The listing builds one solid part. Answer for the finished solid, in the listing's coordinates (mm). A direction names the side the tool comes from. Give positions to 0.01 mm unless a question says otherwise; leave off trailing zeros. Write each loop counter-clockwise with the first axis right and the second up, starting at its lowest first coordinate (ties: lowest second). Pieces come first, ordered by that corner, then holes. Notation, with made-up numbers: (52, 56) -> (106, 56) arc R18 ccw to (106, 77) -> close; hole circle Ø8 at (35, 11). An arc over 180 degrees is marked (long way). One line per question, with ' | ' between items.
Solid Edge part; units mm, degrees
sketch "Sketch1" plane through (0, 0, 0) normal (0, -1, 0) x (1, 0, 0)
  line L0 (8, 6) -> (-8, 6)
  line L1 (-8, 6) -> (-8, -6)
  line L2 (-8, -6) -> (8, -6)
  line L3 (8, -6) -> (8, 6)
extrude "Protrusion1" add sketch "Sketch1" against normal blind 22
sketch "Sketch2" plane through (0, 0, 0) normal (0, -1, 0) x (1, 0, 0)
  line L0 (6, 4) -> (-6, 4)
  line L1 (-6, 4) -> (-6, -4)
  line L2 (-6, -4) -> (6, -4)
  line L3 (6, -4) -> (6, 4)
extrude "Cutout1" cut sketch "Sketch2" against normal blind 20
sketch "Sketch3" plane through (0, 20, 0) normal (0, -1, 0) x (1, 0, 0)
  line L0 (6, -3) -> (2, -3)
  line L1 (2, -3) -> (2, -4)
  line L2 (2, -4) -> (6, -4)
  line L3 (6, -4) -> (6, -3)
  line L4 (6, 3) -> (2.0028, 3)
  line L5 (2.0028, 3) -> (2.0028, 4)
  line L6 (2.0028, 4) -> (6, 4)
  line L7 (6, 4) -> (6, 3)
extrude "LockSideProtrusion" add sketch "Sketch3" along normal blind 19
sketch "Sketch4" plane through (0, 20, 0) normal (0, -1, 0) x (1, 0, 0)
  line L0 (6, 3) -> (6, -3)
  line L1 (6, -3) -> (2.0028, -3)
  line L2 (2.0028, -3) -> (2.0028, 3)
  line L3 (2.0028, 3) -> (6, 3)
extrude "LockBaseProtrusion" add sketch "Sketch4" along normal blind 2
sketch "Sketch5" plane through (4.0014, 18, 0) normal (0, -1, 0) x (1, 0, 0)
  line L0 (-0.0014, 2.48) -> (-0.0014, -2.48)
  line L1 (-0.0014, -2.48) -> (-2.0014, -2.48)
  line L2 (-2.0014, -2.48) -> (-2.0014, 2.48)
  line L3 (-2.0014, 2.48) -> (-0.0014, 2.48)
extrude "LockProtrusion" add sketch "Sketch5" along normal blind 18.07
sketch "Sketch6" plane through (3, -0.07, 0) normal (0, -1, 0) x (1, 0, 0)
  line L0 (-1, -3.93) -> (-1, 3.93)
  line L1 (-1, 3.93) -> (1, 3.93)
  line L2 (1, 3.93) -> (1, -3.93)
  line L3 (1, -3.93) -> (-1, -3.93)
extrude "LockHeadMainProtrusion" add sketch "Sketch6" along normal blind 3
sketch "Sketch7" plane through (3, -0.07, 0) normal (0, -1, 0) x (1, 0, 0)
  line L0 (-3.4, 3.93) -> (-1, 1.53)
  line L1 (-1, 1.53) -> (-1, 3.93)
  line L2 (-1, 3.93) -> (-3.4, 3.93)
  line L3 (-3.4, -3.93) -> (-1, -1.53)
  line L4 (-1, -1.53) -> (-1, -3.93)
  line L5 (-1, -3.93) -> (-3.4, -3.93)
extrude "LockHeadTriangleProtrusion" add sketch "Sketch7" along normal blind 3
sketch "Sketch8" plane through (1.8, -1.57, -3.93) normal (0, 0, -1) x (1, 0, 0)
  line L0 (-2.2, 1.5) -> (0.2, 1.5)
  line L1 (0.2, 1.5) -> (-2.2, -1.5)
  line L2 (-2.2, -1.5) -> (-2.2, 1.5)
extrude "LockHeadTriangleCut" cut sketch "Sketch8" against normal blind 8.6519
sketch "Sketch9" plane through (4, 7.465, 0) normal (1, 0, 0) x (0, 0, 1)
  line L0 (-3.93, 10.535) -> (3.93, 10.535)
  line L1 (3.93, 10.535) -> (3.93, 8.535)
  line L2 (3.93, 8.535) -> (-3.93, 8.535)
  line L3 (-3.93, 8.535) -> (-3.93, 10.535)
extrude "FlapBaseProtrusion" add sketch "Sketch9" along normal blind 4
sketch "Sketch10" plane through (5, -3.07, 0) normal (0, -1, 0) x (1, 0, 0)
  line L0 (3, 3.93) -> (1, 3.93)
  line L1 (1, 3.93) -> (1, -3.93)
  line L2 (1, -3.93) -> (3, -3.93)
  line L3 (3, -3.93) -> (3, 3.93)
extrude "FlapHandleProtrusion" add sketch "Sketch10" along normal blind 2
fillet "SlotInnerRound" radius 1 3 edges at (0, 0, 4) (-6, 0, 0) (0, 0, -4)
fillet "FlapRound" radius 1 3 edges at (6, -5.07, 0) (8, -5.07, 0) (8, -1.07, 0)
sketch "Sketch11" plane through (4, -3.07, 0) normal (0, -1, 0) x (1, 0, 0)
  line L0 (-1.6753, 0.0864) -> (1.042, 1.2263)
  line L1 (1.042, 1.2263) -> (1.042, -1.1917)
  line L2 (1.042, -1.1917) -> (-1.6753, 0.0864)
extrude "MarkCut" cut sketch "Sketch11" against normal blind 0.8
hole "PushHole" at (-2.0513, 20, 0) direction (0, 1, 0) diameter 4 end through all
fillet "LockTriangleRound" radius 1 2 edges at (2, -1.57, 1.53) (2, -1.57, -1.53)
sketch "Sketch12" plane through (8, 11, 0) normal (1, 0, 0) x (0, -1, 0)
  line L0 (-7, 2.48) -> (5, 2.48)
  line L1 (5, 2.48) -> (5, -2.48)
  line L2 (5, -2.48) -> (-7, -2.48)
  line L3 (-7, -2.48) -> (-7, 2.48)
extrude "Cutout2" cut sketch "Sketch12" against normal blind 2
Item 1: A tool of negligible diameter and unlimited length cuts with its end or side. For faces 4 (the face through (0, 11, 6)), 5 (the face through (4, -3.07, -1)), 6 (the face through (4, 10, 3)), 7 (the face through (5, -1.07, 0)), 8 (the face through (4, -2.27, 0)), from which of +Z, -Z, +X, -X, +Y, -Y can it reach the whole face along a straight path? Write none if from no direction.
Answers below:
face 4: +Z, +X, -X, +Y, -Y | face 5: +Z, -Z, -X, -Y | face 6: none | face 7: +Z, -Z, +X | face 8: -Y
Item 2: Find section A-A (y = 2.25). Write down the section's boundary in (x, z).
Answers below:
outline: (-8, -6) -> (8, -6) -> (8, 6) -> (-8, 6) -> close; (2, -2.48) -> (4, -2.48) -> (4, 2.48) -> (2, 2.48) -> close; hole (-6, -4) -> (2, -4) -> (2, -3) -> (6, -3) -> (6, 3) -> (2, 3) -> (2, 4) -> (-6, 4) -> close
Item 3: Find section C-C (y = 9). Write down the section's boundary in (x, z).
Answers below:
outline: (-8, -6) -> (8, -6) -> (8, -2.48) -> (6, -2.48) -> (6, -3) -> (2, -3) -> (2, -4) -> (-6, -4) -> (-6, 4) -> (2, 4) -> (2, 3) -> (6, 3) -> (6, 2.48) -> (8, 2.48) -> (8, 6) -> (-8, 6) -> close; (2, -2.48) -> (4, -2.48) -> (4, 2.48) -> (2, 2.48) -> close
Item 4: Find section D-D (z = -0.5). Count the separate pieces of the cut face and the enclosed holes in it, then the cut area to 3 significant figures.
Answers below:
separate pieces: 3 | enclosed holes: 0 | area: 140 mm²
Item 5: Find section B-B (x = 0.5). Write down the section's boundary in (y, z) (3 decimals).
Answers below:
outline: (-1.195, -3.93) -> (-0.07, -3.93) -> (-0.07, -3.03) -> (-1.195, -3.03) -> close; (-1.195, 3.03) -> (-0.07, 3.03) -> (-0.07, 3.93) -> (-1.195, 3.93) -> close; (0, -6) -> (22, -6) -> (22, 6) -> (0, 6) -> (0, 5) arc R1 ccw to (1, 4) -> (20, 4) -> (20, -4) -> (1, -4) arc R1 ccw to (0, -5) -> close
Item 6: Determine the mould class of faces 1 (the face through (0, 11, -6)), 2 (the face through (3.664, -2.676, 0.648)), 3 (the face through (2, -0.07, -3)) for opening direction Z: pulls with the +Z half, pulls with the -Z half, needs draft (parallel to the pull), parting line crosses it, or undercut.
Answers below:
face 1: pulls with the -Z half | face 2: undercut | face 3: needs draft
Item 7: Consider line 1 (Z direction, x = -3.5, y = 11.75); line 2 (X direction, y = 13, z = 1.5); line 3 (Y direction, x = 4.75, z = -3.25). Determine where each line is inside the solid, lowest interval first. Write a range as [from, to].
Answers below:
line 1: [-6, -4], [4, 6] | line 2: [-8, -6], [2, 4] | line 3: [-3.07, -1.07], [1, 22]
Item 8: Flat-ended cylindrical pins translate along their axes: pin 1 (6.5 mm diameter, centred on x = -2.05, z = 0, fed in from -Y); pin 2 (6.5 mm diameter, centred on x = 4.5, z = 1.5, fed in from -Y); pin 3 (4.5 mm diameter, centred on x = 3, z = -0.5, fed in from -Y). Find the tip coordinate at first contact, or state that the pin passes through.
Answers below:
pin 1: y = 20 | pin 2: y = -5.07 | pin 3: y = -3.07
